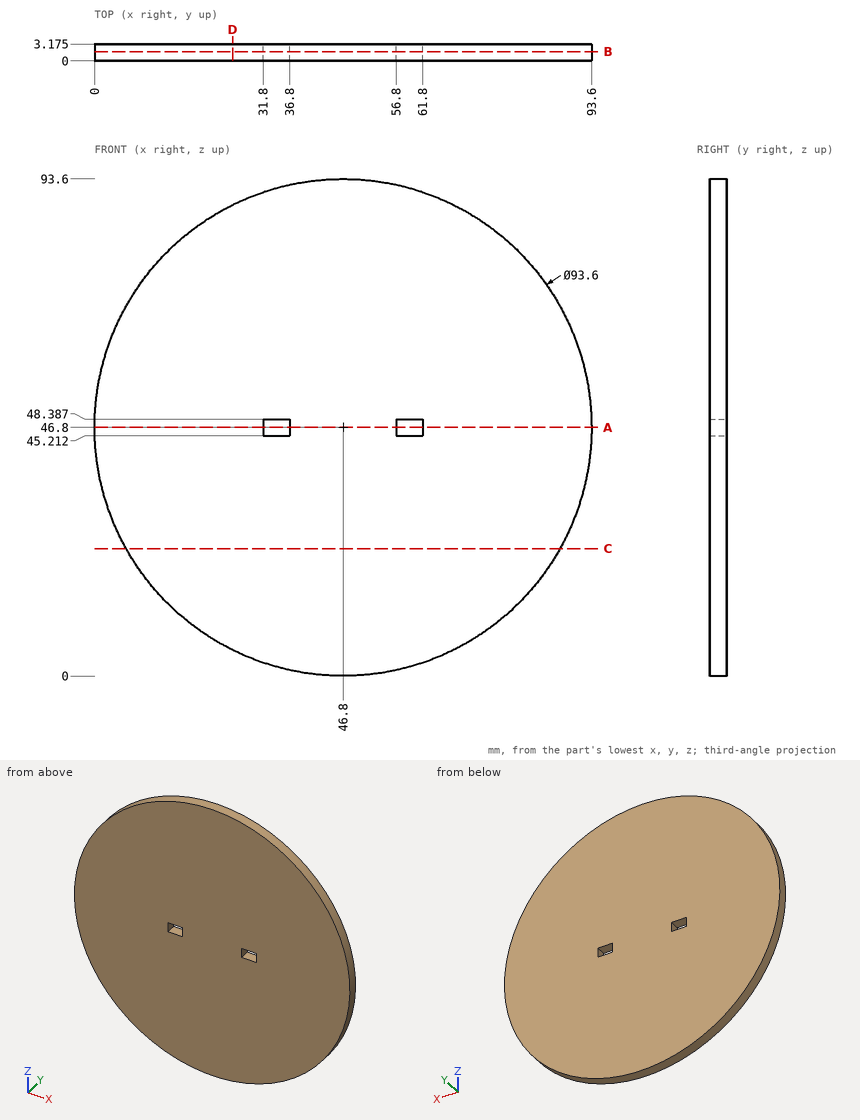
Can you work these out from the drawing? Everything is in mm from the part's minimum corner. Round coordinates to 2 decimals unless told otherwise and drop trailing zeros. Order: outer loops, then holes, each group sorted by start corner. A loop starts at its lowest first (then second) coordinate and runs counter-clockwise, first axis right, second up. Notation, with made-up numbers: (52.25, -27.5) - (110.25, -27.5) arc R25 cw to (110.25, -12.5) - close; hole circle Ø5 at (67, 53). An arc over 180 degrees is marked (long way). Answer in a Markdown table with one row per item.
(1) Suppose I cut it at C-C, the plane z = 24. Please give me the cut outline in (x, y) (1 decimal).
From the geometry:
| item | result |
|---|---|
| outline | (5.9, 0) - (87.7, 0) - (87.7, 3.2) - (5.9, 3.2) - close |
(2) Suppose I cut it at D-D, the plane x = 26. Please give me the cut outline in (y, z) (1 decimal), plus the area to 3 significant figures.
From the geometry:
| item | result |
|---|---|
| outline | (0, 4.9) - (3.2, 4.9) - (3.2, 88.7) - (0, 88.7) - close |
| area | 266 mm2 |
(3) Please list where these lines run through material, in increasing order: L1, parallel to Z at x = 60.5, y = 2.5; L2, parallel to Z at x = 36, y = 1.7; L3, parallel to X at y = 0.9, z = 49. Write a range as from..to.
From the geometry:
| item | result |
|---|---|
| L1 | z = 2.05..45.21, 48.39..91.55 |
| L2 | z = 1.26..45.21, 48.39..92.34 |
| L3 | x = 0.05..93.55 |
(4) For P1, Ø1.6, axis at x = 33.5, y = 2, coming from the +Z side; P2, Ø1.6, axis at x = 33.5, y = 2, coming from the -Z side; P3, Ø1.6, axis at y = 1.5, z = 46, coming from the +X side, each with a flat end and sliding along its axis, tell me the tip position at first contact or that it passes through.
From the geometry:
| item | result |
|---|---|
| P1 | stops at z = 91.9 |
| P2 | stops at z = 1.7 |
| P3 | stops at x = 93.6 |
(5) Suppose I cut it at B-B, the plane y = 1.75. Please give me the cut outline in (x, z).
From the geometry:
| item | result |
|---|---|
| outline | circle Ø93.6 at (46.8, 46.8); hole (31.8, 45.21) - (36.8, 45.21) - (36.8, 48.39) - (31.8, 48.39) - close; hole (56.8, 45.21) - (61.8, 45.21) - (61.8, 48.39) - (56.8, 48.39) - close |
(6) Suppose I cut it at A-A, the plane z = 46.8. Please give me the cut outline in (x, y) (1 decimal).
From the geometry:
| item | result |
|---|---|
| outline | (0, 0) - (31.8, 0) - (31.8, 3.2) - (0, 3.2) - close; (36.8, 0) - (56.8, 0) - (56.8, 3.2) - (36.8, 3.2) - close; (61.8, 0) - (93.6, 0) - (93.6, 3.2) - (61.8, 3.2) - close |
